Geometry: final body of the model. Coordinates: model frame, mm. A direction names the side the tool comes from. Round coordinates to 2 decimals unless told otherwise and drop trailing zeros. Loops run counter-clockwise (first coordinate to the right, second up) from the corner with the lowest first, then second, coordinate; pieces in that order, holes last. Notation, with made-up numbers: (7, 13) -> (22, 13) arc R18 ccw to (22, 19) -> close; hole circle Ø3 at (65.5, 85). An arc over 180 degrees is marked (long way). Answer in a Markdown table with one row per item.
```python
from build123d import *

# Parameters (mm, degrees)
SKETCH1_W           = 14
SKETCH1_H           = 14
BOSS_EXTRUDE1_DEPTH = 75
SKETCH2_R           = 2.5
CUT_EXTRUDE1_DEPTH  = 30
SKETCH3_W           = 14
SKETCH3_H           = 45
BOSS_EXTRUDE2_DEPTH = 14
SKETCH4_W           = 14
SKETCH4_H           = 45
BOSS_EXTRUDE3_DEPTH = 14


with BuildPart() as part:
    # Sketch1 → Boss-Extrude1 (new body)
    with BuildSketch(Plane(origin=(0, 0, 0), x_dir=(1, 0, 0), z_dir=(0, 1, 0))):
        Rectangle(SKETCH1_W, SKETCH1_H)
    extrude(amount=BOSS_EXTRUDE1_DEPTH)

    # Sketch2 → Cut-Extrude1 (cut)
    with BuildSketch(Plane(origin=(0, 75, 0), x_dir=(1, 0, 0), z_dir=(0, 1, 0))):
        Circle(SKETCH2_R)
    extrude(amount=-CUT_EXTRUDE1_DEPTH, mode=Mode.SUBTRACT)

    # Sketch3 → Boss-Extrude2 (add)
    with BuildSketch(Plane(origin=(7, 0, 0), x_dir=(0, 0, -1), z_dir=(1, 0, 0))):
        with Locations((0, 52.5)):
            Rectangle(SKETCH3_W, SKETCH3_H)
    extrude(amount=BOSS_EXTRUDE2_DEPTH)

    # Sketch4 → Boss-Extrude3 (add)
    with BuildSketch(Plane.ZY.offset(7)):
        with Locations((0, 52.5)):
            Rectangle(SKETCH4_W, SKETCH4_H)
    extrude(amount=BOSS_EXTRUDE3_DEPTH)


solid = part.part
```
Item 1: Reachability of faces 1 (the face through (-0.54, 60.21, 2.44)), 2 (the face through (0, 0, 0)), 3 (the face through (14, 30, 0)), 4 (the face through (-14, 30, 0)) from +Z, -Z, +X, -X, +Y, -Y: full face, straight path, thin tool, end or side. Return the list, or none.
Answer:
| item | result |
|---|---|
| face 1 | +Y |
| face 2 | +Z, -Z, +X, -X, -Y |
| face 3 | +Z, -Z, +X, -Y |
| face 4 | +Z, -Z, -X, -Y |
Item 2: Line query: probe 1 along Z at (x, y) = (0, 67.5); probe 2 along X at (y, z) = (53.5, 0); probe 3 along Y at (x, z) = (11.5, 1). Output: solid intervals per line, ascending. Write a range as [from, to].
Answer:
| item | result |
|---|---|
| probe 1 | z = [-7, -2.5], [2.5, 7] |
| probe 2 | x = [-21, -2.5], [2.5, 21] |
| probe 3 | y = [30, 75] |
Item 3: Pin query (flat end, axial travel): pin 1 Ø4 at (x, z) = (-16.5, -3) entering from -Y; pin 2 Ø7 at (y, z) = (19.5, -2) entering from +X; pin 3 Ø4.5 at (x, z) = (0, 0) entering from +Y. Return the tip coordinate at first contact, or that it passes through.
Answer:
| item | result |
|---|---|
| pin 1 | stops at y = 30 |
| pin 2 | stops at x = 7 |
| pin 3 | stops at y = 45 |
Item 4: Cut plane C-C (y = 52). Output: boundary loops of the cut face in (x, z), then the cut area to 3 significant figures.
Answer:
| item | result |
|---|---|
| outline | (-21, -7) -> (21, -7) -> (21, 7) -> (-21, 7) -> close; hole circle Ø5 at (0, 0) |
| area | 568 mm² |
Item 5: Cut plane A-A (z = 0). Output: boundary loops of the cut face in (x, y), then the cut area to 3 significant figures.
Answer:
| item | result |
|---|---|
| outline | (-21, 30) -> (-7, 30) -> (-7, 0) -> (7, 0) -> (7, 30) -> (21, 30) -> (21, 75) -> (2.5, 75) -> (2.5, 45) -> (-2.5, 45) -> (-2.5, 75) -> (-21, 75) -> close |
| area | 2,160 mm² |
Item 6: Cut plane D-D (z = 6). Output: boundary loops of the cut face in (x, y), then the cut area to 3 significant figures.
Answer:
| item | result |
|---|---|
| outline | (-21, 30) -> (-7, 30) -> (-7, 0) -> (7, 0) -> (7, 30) -> (21, 30) -> (21, 75) -> (-21, 75) -> close |
| area | 2,310 mm² |
Item 7: Cut plane B-B (x = 0). Output: boundary loops of the cut face in (y, z), then the cut area to 3 significant figures.
Answer:
| item | result |
|---|---|
| outline | (0, -7) -> (75, -7) -> (75, -2.5) -> (45, -2.5) -> (45, 2.5) -> (75, 2.5) -> (75, 7) -> (0, 7) -> close |
| area | 900 mm² |
